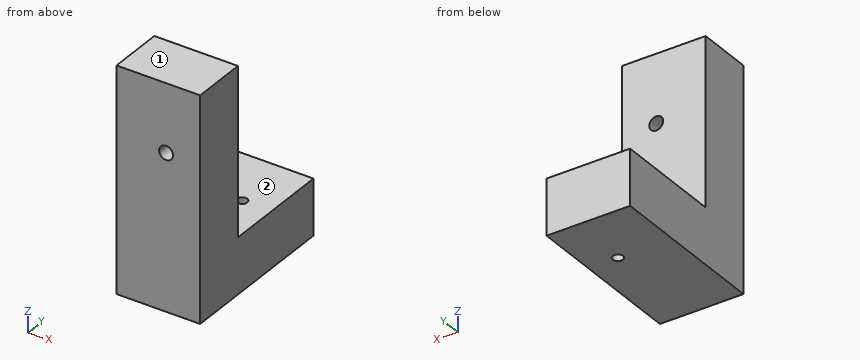
```python
from build123d import *

# Parameters (mm, degrees)
F1_DEPTH = 76.2
F3_D     = 9.525
F5_D     = 12.7


with BuildPart() as f1:
    # F0 (on Right) → F1 (new body)
    with BuildSketch(Plane.YZ):
        Polygon((-152.4, 203.2), (-152.4, 0), (0, 0), (0, 50.8), (-101.6, 50.8), (-101.6, 203.2), align=None)
    extrude(amount=F1_DEPTH)

    # F3 (through all)
    with Locations(Plane.XY.offset(50.8)):
        with Locations((49.338017, -56.317471)):
            Hole(F3_D / 2)

    # F5 (through all)
    with Locations(Plane(origin=(0, -101.6, 0), x_dir=(-1, 0, 0), z_dir=(0, 1, 0))):
        with Locations((-45.108046, 141.260952)):
            Hole(F5_D / 2)


solid = f1.part
```
Can you work these out from the model? Positions are in its coordinate system, mm. Face numbers are marked on the shaded views. A direction names the side the tool comes from. Coordinates: 2 decimals unless noted, no trailing zeros. Loops run counter-clockwise (first coordinate to the right, second up) from the corner with the lowest first, then second, coordinate; pieces in that order, holes last. Notation, with made-up numbers: M 30,59.5 L 53,59.5 A33 cw 53,98.5 Z; hole C -35.5,52 d2. An arc over 180 degrees is marked long. Put each result on its own line as item: value. Start each with the question number.
(1) Imagine slicing it at B-B on z = 170.5. List the corners of the cut face in (x, y) for me.
(2) Imagine slicing it at A-A on x = 28. List the corners of the cut face in (y, z) for me, and give its area (3 significant figures).
(3) I need wall thicknesses on probe 1 along Z at (x, y) = (65.5, -40); probe 2 along Y at (x, z) = (27, 146). Which ranges of each line are inside material? Lowest first, please.
(4) Which directions (+Z, -Z, +X, -X, +Y, -Y) give clear straight access to the entire face, cutting with the end or side of a thin tool? Please do the marked faces 1 and 2.
(5) Will these pins go through, and if not, where does the flat tip stop? pin 1 Ø1.5 at (x, y) = (43, -97) entering from +Z; pin 2 Ø12 at (x, z) = (53, 111) entering from +Y.
(6) Imagine slicing it at C-C on y = -94. List the corners of the cut face in (x, z) for me, and give its area (3 significant figures).
Worked answers:
1. outline: M 0,-152.4 L 76.2,-152.4 L 76.2,-101.6 L 0,-101.6 Z
2. outline: M -152.4,0 L 0,0 L 0,50.8 L -101.6,50.8 L -101.6,203.2 L -152.4,203.2 Z
2. area: 15,500 mm2
3. probe 1: z = 0 to 50.8
3. probe 2: y = -152.4 to -101.6
4. face 1: +Z, +X, -X, +Y, -Y
4. face 2: +Z, +X, -X, +Y
5. pin 1: stops at z = 50.8
5. pin 2: stops at y = -101.6
6. outline: M 0,0 L 76.2,0 L 76.2,50.8 L 0,50.8 Z
6. area: 3,870 mm2
